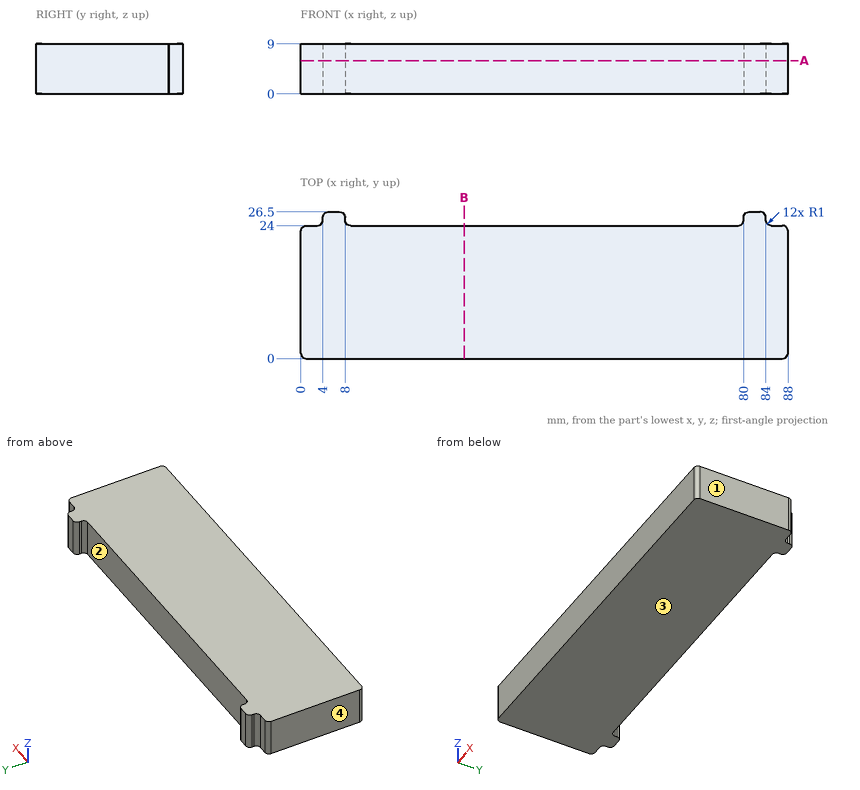
Could you check a few things on this drawing? It's one solid part, dimensions in mm from its lowest x, y, z. Coordinates: 2 decimals unless noted, no trailing zeros. Order: outer loops, then holes, each group sorted by start corner. A loop starts at its lowest first (then second) coordinate and runs counter-clockwise, first axis right, second up.
1) Imagine slicing it at A-A on z = 6. List the corners of the cut face in (x, y) for me, and give its area (3 significant figures).
2) Imagine slicing it at B-B on x = 29.5. List the corners of the cut face in (y, z) for me.
3) I need wall thicknesses on line 1 (Y direction, x = 59.5, z = 8.75); line 2 (Y direction, x = 8.5, z = 3.5). Which ranges of each line are inside material? Lowest first, please.
4) Will these pins go through, and if not, where does the flat tip stop? pin 1 (1.6 mm diameter, centred on x = 86, z = 3.5, fed in from +Y); pin 2 (0.6 mm diameter, centred on y = 25.5, z = 6, fed in from +X).
5) We'd pull the mould along X, two halves only. Please class the marked faces 1, 2, 3 and 4: +X half, -X half, draft (parallel to the pull), parting line (faces both ways), or undercut.
Response values:
1. outline: (0, 1) arc R1 ccw to (1, 0) - (87, 0) arc R1 ccw to (88, 1) - (88, 23) arc R1 ccw to (87, 24) - (85, 24) arc R1 cw to (84, 25) - (84, 25.5) arc R1 ccw to (83, 26.5) - (81, 26.5) arc R1 ccw to (80, 25.5) - (80, 25) arc R1 cw to (79, 24) - (9, 24) arc R1 cw to (8, 25) - (8, 25.5) arc R1 ccw to (7, 26.5) - (5, 26.5) arc R1 ccw to (4, 25.5) - (4, 25) arc R1 cw to (3, 24) - (1, 24) arc R1 ccw to (0, 23) - close
1. area: 2,130 mm2
2. outline: (0, 0) - (24, 0) - (24, 9) - (0, 9) - close
3. line 1: y = 0 to 24
3. line 2: y = 0 to 24.13
4. pin 1: stops at y = 24
4. pin 2: stops at x = 84
5. face 1: +X half
5. face 2: undercut
5. face 3: draft
5. face 4: -X half
